Source: three-view drawing plus pictorial views. Frame: mm from the lowest corner of the part. Coordinates: 2 decimals unless noted, no trailing zeros. Order: outer loops, then holes, each group sorted by start corner. A loop starts at its lowest first (then second) coordinate and runs counter-clockwise, first axis right, second up. Notation, with made-up numbers: (-39.75, 23) -> (-32.75, 23) arc R16 ccw to (-32.75, 37) -> close; hole circle Ø3 at (77, 88.25). An arc over 180 degrees is marked (long way). Use CSV: the item, a comma, the result in double quotes. Start each with the question number.
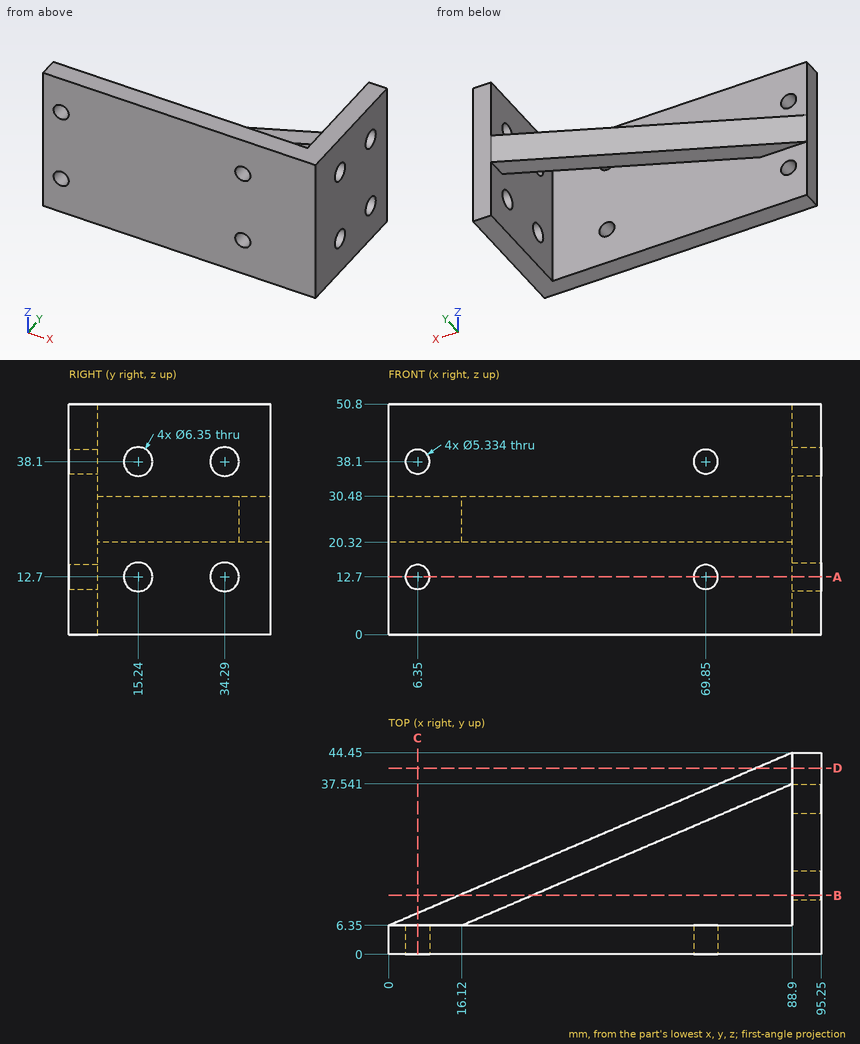
1. Section C-C on x = 6.35. Return loops of the section in (y, z).
2. Section A-A on z = 12.7. State how many separate pieces and enclosed holes the cut face has.
3. Material intervals for line 1 along X through (y, z) = (2, 12.5); line 2 along X through (y, z) = (4, 12); line 3 along X through (y, z) = (13, 7), sorted ascending.
4. Section B-B on y = 13. Return loops of the section in (x, z).
5. Contact query for flat-ended pins moving along their axis: P1, Ø7.5, axis at y = 15.24, z = 38.1, coming from the -X side; P2, Ø5, axis at x = 69.85, z = 38.1, coming from the -Y side; P3, Ø10, axis at y = 25, z = 23, coming from the -X side; P4, Ø19, axis at x = 41, y = 25, coming from the +Z side. Output: stop coordinate, or through.
6. Section D-D on y = 41. Return loops of the section in (x, z), then the cut area to 3 significant figures.
Values follow:
1,outline,"(0, 0) -> (6.35, 0) -> (6.35, 10.03) -> (0, 10.03) -> close; (0, 15.37) -> (6.35, 15.37) -> (6.35, 20.32) -> (9.07, 20.32) -> (9.07, 30.48) -> (6.35, 30.48) -> (6.35, 35.43) -> (0, 35.43) -> close; (0, 40.77) -> (6.35, 40.77) -> (6.35, 50.8) -> (0, 50.8) -> close"
2,separate pieces,"5"
2,enclosed holes,"0"
3,line 1,"x = 0 to 3.69, 9.01 to 67.19, 72.51 to 95.25"
3,line 2,"x = 0 to 3.78, 8.92 to 67.28, 72.42 to 95.25"
3,line 3,"x = 88.9 to 95.25"
4,outline,"(15.52, 20.32) -> (31.64, 20.32) -> (31.64, 30.48) -> (15.52, 30.48) -> close; (88.9, 0) -> (95.25, 0) -> (95.25, 10.45) -> (88.9, 10.45) -> close; (88.9, 14.95) -> (95.25, 14.95) -> (95.25, 35.85) -> (88.9, 35.85) -> close; (88.9, 40.35) -> (95.25, 40.35) -> (95.25, 50.8) -> (88.9, 50.8) -> close"
5,P1,"stops at x = 88.9"
5,P2,"passes through"
5,P3,"stops at x = 31.85"
5,P4,"stops at z = 30.48"
6,outline,"(80.85, 20.32) -> (88.9, 20.32) -> (88.9, 0) -> (95.25, 0) -> (95.25, 50.8) -> (88.9, 50.8) -> (88.9, 30.48) -> (80.85, 30.48) -> close"
6,area,"404 mm2"
